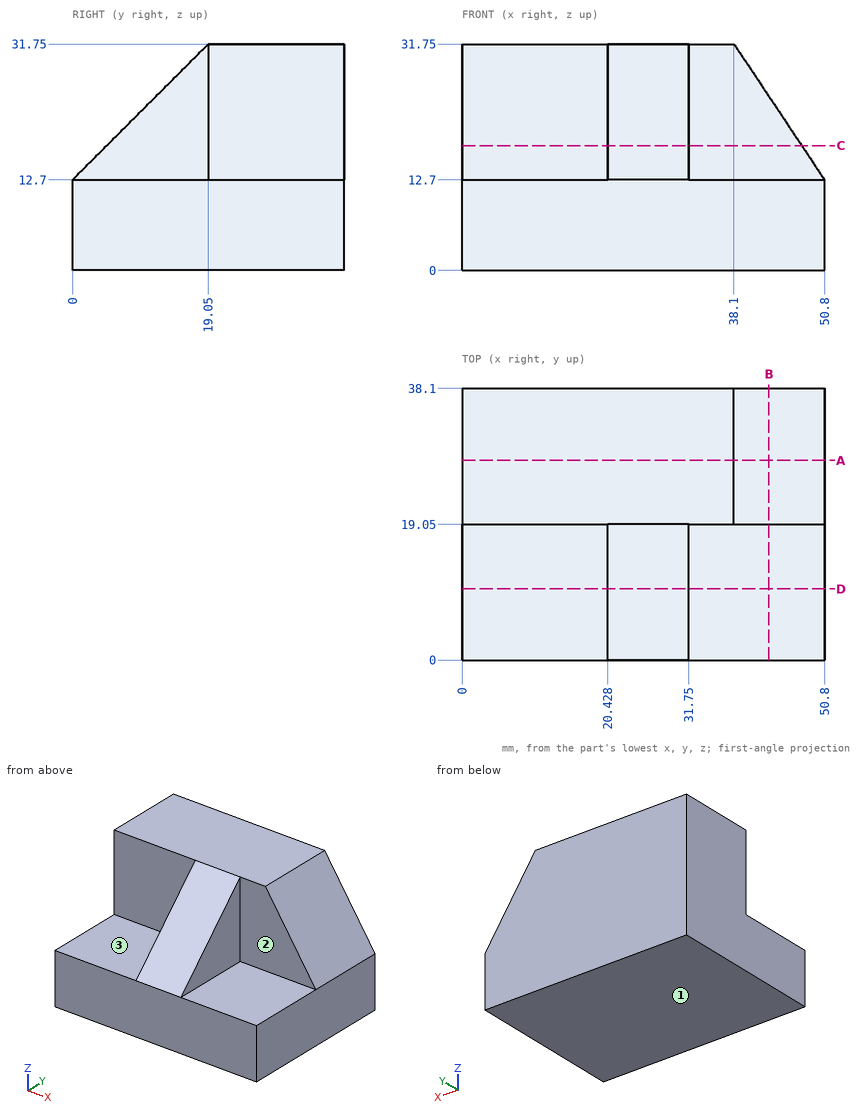
Could you check a few things on this drawing? It's one solid part, dimensions in mm from its lowest x, y, z. A direction names the side the tool comes from. Give positions to 0.01 mm unless a question says otherwise; leave off trailing zeros. Order: outer loops, then holes, each group sorted by start corner. A loop starts at its lowest first (then second) coordinate and runs counter-clockwise, first axis right, second up. Notation, with made-up numbers: (77, -14.5) - (107, -14.5) arc R22 cw to (107, 23.5) - close; hole circle Ø4 at (-34.75, 83). An arc over 180 degrees is marked (long way). Answer as a JSON object with one key per item and string values. Group by question number.
Item 1: Which directions (+Z, -Z, +X, -X, +Y, -Y) give clear straight access to the entire face, cutting with the end or side of a thin tool? Please do the marked faces 1, 2 and 3.
Item 2: If we section it at D-D on y = 10: Please give me the cut outline in (x, z), and give its area (3 significant figures).
Item 3: If we section it at B-B on x = 43: Please give me the cut outline in (y, z).
Item 4: For P1, Ø9.5, axis at x = 40.5, y = 7.5, coming from the +Z side; P2, Ø5.5, axis at x = 15, z = 23, coming from the -Y side; P3, Ø15, axis at x = 14, y = 6.5, coming from the +Z side; P4, Ø5.5, axis at y = 7.5, z = 25.5, coming from the +X side, each with a flat end and sliding along its axis, tell me the tip position at first contact or that it passes through.
Item 5: If we section it at C-C on z = 17.5: Please give me the cut outline in (x, y).
Item 6: If we section it at A-A on y = 28: Please give me the cut outline in (x, z).
Item 7: Please list where these lines run through material, in increasing order: probe 1 along X at (y, z) = (2.5, 15); probe 2 along Y at (x, z) = (44.5, 16); probe 3 along Z at (x, y) = (34, 2).
Result set:
{
 "1": {"face 1": "-Z, +X, -X, +Y, -Y", "face 2": "+Z, +X, -Y", "face 3": "+Z, -X, -Y"},
 "2": {"outline": "(0, 0) - (50.8, 0) - (50.8, 12.7) - (31.75, 12.7) - (31.75, 22.7) - (20.43, 22.7) - (20.43, 12.7) - (0, 12.7) - close", "area": "758 mm²"},
 "3": {"outline": "(0, 0) - (38.1, 0) - (38.1, 24.4) - (19.05, 24.4) - (19.05, 12.7) - (0, 12.7) - close"},
 "4": {"P1": "z = 12.7", "P2": "y = 19.05", "P3": "z = 23.06", "P4": "through"},
 "5": {"outline": "(0, 19.05) - (20.43, 19.05) - (20.43, 4.8) - (31.75, 4.8) - (31.75, 19.05) - (47.6, 19.05) - (47.6, 38.1) - (0, 38.1) - close"},
 "6": {"outline": "(0, 0) - (50.8, 0) - (50.8, 12.7) - (38.1, 31.75) - (0, 31.75) - close"},
 "7": {"probe 1": "20.43 to 31.75", "probe 2": "19.05 to 38.1", "probe 3": "0 to 12.7"}
}
